from build123d import *

# Parameters (mm, degrees)
F0_R      = 9.25
F0_R_2    = 7.75
F1_DEPTH  = 12
F2_R      = 9.75
F2_R_2    = 7.25
F3_DEPTH  = 2.5
F4_R      = 10.75
F4_R_2    = 7.25
F5_DEPTH  = 4.5
F6_SIZE   = 2
F7_R      = 7.5767654437
F7_R_2    = 7.25
F8_DEPTH  = 1
F9_R      = 8.25
F9_R_2    = 7.5767654437
F9_R_3    = 7.25
F10_DEPTH = 0.5
F11_SIZE  = 0.1


with BuildPart() as f1:
    # F0 (on Front) → F1 (new body)
    with BuildSketch(Plane.XZ):
        Circle(F0_R)
        Circle(F0_R_2, mode=Mode.SUBTRACT)
    extrude(amount=F1_DEPTH)

    # F2 (on face) → F3 (join)
    with BuildSketch(Plane.XZ.offset(12)):
        Circle(F2_R)
        Circle(F2_R_2, mode=Mode.SUBTRACT)
    extrude(amount=F3_DEPTH)

    # F4 (on face) → F5 (join)
    with BuildSketch(Plane.XZ.offset(14.5)):
        Circle(F4_R)
        Circle(F4_R_2, mode=Mode.SUBTRACT)
    extrude(amount=F5_DEPTH)

    # F6
    f6_edges = [f1.edges().sort_by_distance(p)[0] for p in [
        (-10.75, -19, 0),
    ]]
    chamfer(f6_edges, length=F6_SIZE)

    # F7 (on face) → F8 (join)
    with BuildSketch(Plane.XZ.offset(19)):
        Circle(F7_R)
        Circle(F7_R_2, mode=Mode.SUBTRACT)
    extrude(amount=F8_DEPTH)

    # F9 (on face) → F10 (join)
    with BuildSketch(Plane.XZ.offset(20)):
        Circle(F9_R)
        Circle(F9_R_2, mode=Mode.SUBTRACT)
        Circle(F9_R_2)
        Circle(F9_R_3, mode=Mode.SUBTRACT)
    extrude(amount=F10_DEPTH)

    # F11
    f11_edges = [f1.edges().sort_by_distance(p)[0] for p in [
        (-7.25, -20.5, 0),
        (-8.25, -20.5, 0),
    ]]
    chamfer(f11_edges, length=F11_SIZE)


solid = f1.part
Design review of the part built by this model. Coordinates are the model's own, in mm. A direction names the side the tool comes from. Coordinates: 2 decimals unless noted, no trailing zeros. Loops run counter-clockwise (first coordinate to the right, second up) from the corner with the lowest first, then second, coordinate; pieces in that order, holes last.
Item 1: For faces 1 (the cylindrical face through (-2.01, -5.92, -9.03)), 2 (the cylindrical face through (7.62, -20.2, -3.16)), 3 (the cylindrical face through (-0.99, -19.49, 7.51)), list the 3-axis set-ups (+Z, -Z, +X, -X, +Y, -Y) from which the entire face can be reached by the end or side of a thin tool; tool diameter is ignored.
Completed:
face 1: +Y
face 2: -Y
face 3: none
Item 2: Draft analysis for pull direction Y (two halves, no side actions). For faces 4 (the flat face through (-7, -19, 4)), 5 (the cylindrical face through (3.35, -16.14, -6.43)), 6 (the flat face through (2, -14.5, -10)), state which applies: pulls with the +Y half, pulls with the -Y half, needs draft (parallel to the pull), parting line crosses it, or undercut.
Completed:
face 4: undercut
face 5: needs draft
face 6: pulls with the +Y half
Item 3: Clearance check with flat-ended pins moving along their axes: pin 1 (8 mm diameter, centred on x = 2, z = 0.5, fed in from +Y); pin 2 (8 mm diameter, centred on x = 3.5, z = -0.5, fed in from +Y); pin 3 (5 mm diameter, centred on x = 6, z = 7.5, fed in from +Y); pin 4 (1 mm diameter, centred on x = -8, z = -5.5, fed in from -Y). State where each tip first meets the part, or that it passes through.
Completed:
pin 1: passes through
pin 2: stops at y = -12
pin 3: stops at y = 0
pin 4: stops at y = -18.54
Item 4: Add section C-C (y = -3.25). Write out the cut boundary in (x, z).
Completed:
outline: circle Ø18.5 at (0, 0); hole circle Ø15.5 at (0, 0)
Item 5: Wall thickness on L1, parallel to Z at x = 0, y = -4.75; L2, parallel to X at y = -10.25, z = -5.5; L3, parallel to Z at x = -6.25, y = -6.75: over which ranges is each line inside the solid? List them lowest first.
Completed:
L1: z = -9.25 to -7.75, 7.75 to 9.25
L2: x = -7.44 to -5.46, 5.46 to 7.44
L3: z = -6.82 to -4.58, 4.58 to 6.82
